Here's the drawing with two shaded views (mm, measured from the low corner). I have some questions. Round coordinates to 2 decimals unless told otherwise and drop trailing zeros. Loops run counter-clockwise (first coordinate to the right, second up) from the corner with the lowest first, then second, coordinate; pieces in that order, holes last. Notation, with made-up numbers: (40, -22) -> (52, -22) arc R18 cw to (52, -6) -> close; hole circle Ø8 at (11, 54). An arc over 180 degrees is marked (long way). Use a Markdown table: item, result.
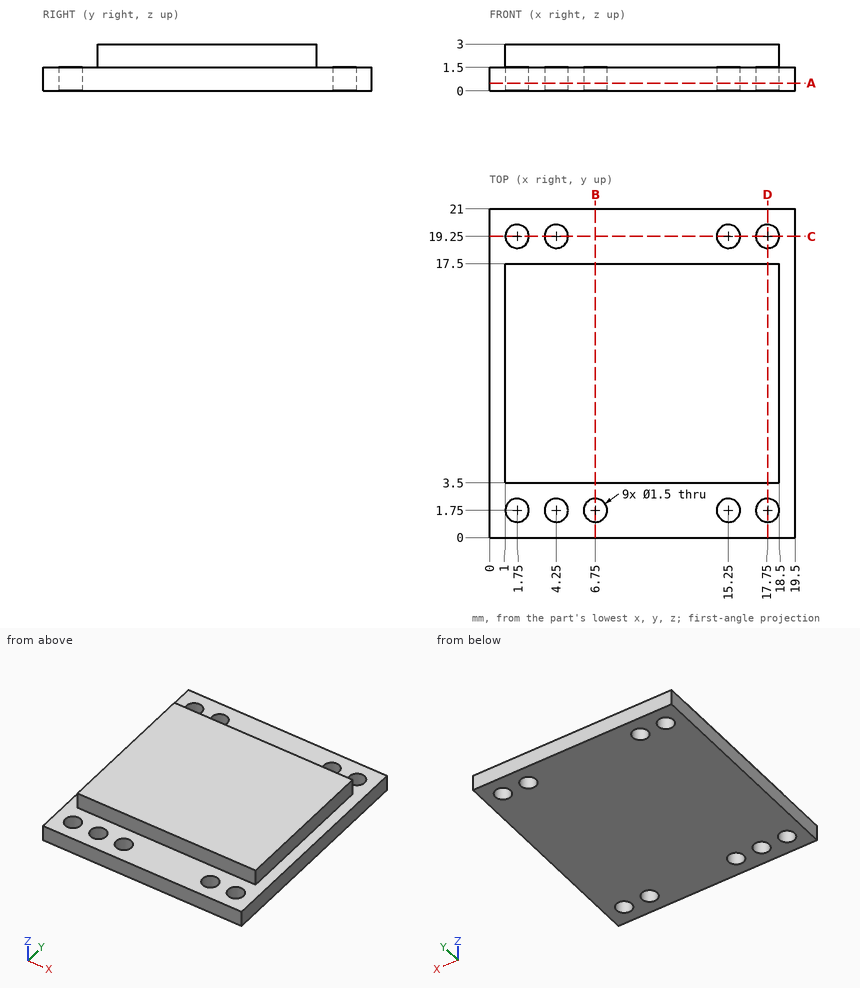
1. I want a section at D-D (x = 17.75). Please give me the cut outline in (y, z), plus the area to 3 significant figures.
Answer sheet:
| item | result |
|---|---|
| outline | (0, 0) -> (1, 0) -> (1, 1.5) -> (0, 1.5) -> close; (2.5, 0) -> (18.5, 0) -> (18.5, 1.5) -> (17.5, 1.5) -> (17.5, 3) -> (3.5, 3) -> (3.5, 1.5) -> (2.5, 1.5) -> close; (20, 0) -> (21, 0) -> (21, 1.5) -> (20, 1.5) -> close |
| area | 48.0 mm² |
2. I want a section at B-B (x = 6.75). Please give me the cut outline in (y, z), plus the area to 4 significant figures.
Answer sheet:
| item | result |
|---|---|
| outline | (0, 0) -> (1, 0) -> (1, 1.5) -> (0, 1.5) -> close; (2.5, 0) -> (21, 0) -> (21, 1.5) -> (17.5, 1.5) -> (17.5, 3) -> (3.5, 3) -> (3.5, 1.5) -> (2.5, 1.5) -> close |
| area | 50.25 mm² |
3. I want a section at C-C (y = 19.25). Please give me the cut outline in (x, z).
Answer sheet:
| item | result |
|---|---|
| outline | (0, 0) -> (1, 0) -> (1, 1.5) -> (0, 1.5) -> close; (2.5, 0) -> (3.5, 0) -> (3.5, 1.5) -> (2.5, 1.5) -> close; (5, 0) -> (14.5, 0) -> (14.5, 1.5) -> (5, 1.5) -> close; (16, 0) -> (17, 0) -> (17, 1.5) -> (16, 1.5) -> close; (18.5, 0) -> (19.5, 0) -> (19.5, 1.5) -> (18.5, 1.5) -> close |
4. I need wall thicknesses on line 1 (Y direction, x = 1.75, z = 0.75); line 2 (Y direction, x = 6.75, z = 0.85); line 3 (Z direction, x = 12.5, y = 1.5). Which ranges of each line are inside material? Lowest first, please.
Answer sheet:
| item | result |
|---|---|
| line 1 | y = 0 to 1, 2.5 to 18.5, 20 to 21 |
| line 2 | y = 0 to 1, 2.5 to 21 |
| line 3 | z = 0 to 1.5 |
5. Will these pins go through, and if not, where does the flat tip stop? pin 1 Ø1.6 at (x, z) = (13.5, 2.5) entering from -Y; pin 2 Ø1.7 at (x, y) = (4.25, 1.75) entering from +Z.
Answer sheet:
| item | result |
|---|---|
| pin 1 | stops at y = 3.5 |
| pin 2 | stops at z = 1.5 |
6. I want a section at A-A (z = 0.5). State how many separate pieces and enclosed holes the cut face has, plus the area to 3 significant figures.
Answer sheet:
| item | result |
|---|---|
| separate pieces | 1 |
| enclosed holes | 9 |
| area | 394 mm² |
